Here's how the part is built. I have some questions about the finished solid (model axes, mm). A direction names the side the tool comes from. Round coordinates to 2 decimals unless told otherwise and drop trailing zeros. Order: outer loops, then holes, each group sorted by start corner. A loop starts at its lowest first (then second) coordinate and runs counter-clockwise, first axis right, second up. Notation, with made-up numbers: (-25, 47.5) - (29, 47.5) arc R22 cw to (29, 75.5) - close; hole circle Ø1 at (56.5, -38). An arc over 180 degrees is marked (long way). Answer as a JSON object with one key per item and string values.
```python
from build123d import *

# Parameters (mm, degrees)
BOSS_EXTRUDE1_DEPTH        = 100
CHAMFER1_SIZE              = 0.5
SKETCH5_R                  = 2
CUT_EXTRUDE1_DEPTH         = 200
CHAMFER2_SIZE              = 0.5
LPATTERN1_COUNT            = 3
LPATTERN1_PITCH            = 35
CHAMFER2_OF_LPATTERN1_SIZE = 0.5
CUT_EXTRUDE2_DEPTH         = 10
CUT_EXTRUDE2_DEPTH_BACK    = 10
SKETCH6_W                  = 15
SKETCH6_H                  = 40


with BuildPart() as part:
    # Sketch1 → Boss-Extrude1 (new body)
    with BuildSketch(Plane.XY):
        with BuildLine():
            Line((-3, 2), (-5, 2))
            Line((-5, 2), (-5, -2))
            Line((-5, -2), (5, -2))
            Line((5, -2), (5, 2))
            Line((5, 2), (3, 2))
            Line((3, 2), (3, 1.25))
            ThreePointArc((3, 1.25), (3.530330086, 1.030330086), (3.75, 0.5))
            ThreePointArc((3.75, 0.5), (3.530330086, -0.030330086), (3, -0.25))
            Line((3, -0.25), (3, -1))
            Line((3, -1), (-3, -1))
            Line((-3, -1), (-3, -0.25))
            ThreePointArc((-3, -0.25), (-3.75, 0.5), (-3, 1.25))
            Line((-3, 1.25), (-3, 2))
        make_face()
    extrude(amount=BOSS_EXTRUDE1_DEPTH)

    # Chamfer1
    chamfer1_edges = [part.edges().sort_by_distance(p)[0] for p in [
        (-3, -1, 50),
        (3, -1, 50),
        (5, 2, 50),
        (5, -2, 50),
        (-5, -2, 50),
        (-5, 2, 50),
    ]]
    chamfer(chamfer1_edges, length=CHAMFER1_SIZE)

    # Sketch5 → Cut-Extrude1 (cut)
    with BuildSketch(Plane(origin=(0, -1, 0), x_dir=(1, 0, 0), z_dir=(0, 1, 0))):
        with Locations(Location((0, -10, 0), (0, 0, 270))):
            Circle(SKETCH5_R)
        with Locations(Location((0, -20, 0), (0, 0, 270))):
            Circle(SKETCH5_R)
    cut_extrude1 = extrude(amount=-CUT_EXTRUDE1_DEPTH, mode=Mode.SUBTRACT)

    # Chamfer2
    chamfer2_edges = [part.edges().sort_by_distance(p)[0] for p in [
        (0, -1, 8),
        (0, -1, 18),
    ]]
    chamfer(chamfer2_edges, length=CHAMFER2_SIZE - 0.0001)  # a hair under: the kernel refuses the full size

    # LPattern1: Cut-Extrude1 ×3
    with Locations(*[(0, 0, i * LPATTERN1_PITCH) for i in range(1, LPATTERN1_COUNT)]):
        add(cut_extrude1, mode=Mode.SUBTRACT)

    # Chamfer2 of LPattern1
    chamfer2_of_lpattern1_edges = [part.edges().sort_by_distance(p)[0] for p in [
        (0, -1, 43),
        (0, -1, 53),
        (0, -1, 78),
        (0, -1, 88),
    ]]
    chamfer(chamfer2_of_lpattern1_edges, length=CHAMFER2_OF_LPATTERN1_SIZE - 0.0001)  # a hair under: the kernel refuses the full size

    # Sketch6 → Cut-Extrude2 (cut, two sides: drawn at the far end of the back side and taken through both)
    with BuildSketch(Plane(origin=(0, 0, 0), x_dir=(1, 0, 0), z_dir=(0, 1, 0)).offset(-CUT_EXTRUDE2_DEPTH_BACK)):
        with Locations((0, -80)):
            Rectangle(SKETCH6_W, SKETCH6_H)
    extrude(amount=CUT_EXTRUDE2_DEPTH + CUT_EXTRUDE2_DEPTH_BACK, mode=Mode.SUBTRACT)


solid = part.part
```
1. Imagine slicing it at C-C (z = 50). List the corners of the cut face in (x, y) for me.
Responses:
{"outline": "(-5, -1.5) - (-4.5, -2) - (4.5, -2) - (5, -1.5) - (5, 1.5) - (4.5, 2) - (3, 2) - (3, 1.25) arc R0.75 cw to (3, -0.25) - (3, -0.5) - (2.5, -1) - (-2.5, -1) - (-3, -0.5) - (-3, -0.25) arc R0.75 cw to (-3, 1.25) - (-3, 2) - (-4.5, 2) - (-5, 1.5) - close"}
2. If I drill on L1, parallel to X at y = 0.4, z = 42.5; L2, parallel to Y at x = 1.5, z = 51; L3, parallel to X at y = 1.1, z = 11, over which ranges is the centre line in solid material (lowest first)? Write a range as [from, to].
Responses:
{"L1": "[-5, -3.74], [3.74, 5]", "L2": "[-2, -1]", "L3": "[-5, -3.45], [3.45, 5]"}
3. Thinking about a two-plate mould opening in X: for faces 4 (the face through (0.601, -1.746, 56.908)), 5 (the face through (-0.1, -1.4, 60)), 6 (the face through (-0.766, -1.746, 46.847)), 7 (the face through (5, 0, 30)), which applies, pulls with the +X half, pulls with the -X half, needs draft (parallel to the pull), parting line crosses it, or undercut?
Responses:
{"face 4": "undercut", "face 5": "needs draft", "face 6": "undercut", "face 7": "pulls with the +X half"}
4. For faces 1 (the face through (4, 2, 30)), 2 (the face through (0, -1, 30)), 3 (the face through (-3.75, 0.48, 29.58)), which set-ups out of +Z, -Z, +X, -X, +Y, -Y let a thin tool reach every point of the face, with its end or its side?
Responses:
{"face 1": "+Z, -Z, +X, -X, +Y", "face 2": "+Z, -Z, +Y", "face 3": "+Z, -Z"}
5. For P1, Ø2.5, axis at x = 0, z = 10, coming from the +Y side; P2, Ø4, axis at x = 0, z = 23, coming from the +Y side, each with a flat end and sliding along its axis, tell me the tip position at first contact or that it passes through.
Responses:
{"P1": "through", "P2": "y = -1"}
6. Imagine slicing it at A-A (x = 0). List the corners of the cut face in (y, z) for me.
Responses:
{"outline": "(-2, 0) - (-1, 0) - (-1, 7.5) - (-1.5, 8) - (-2, 8) - close; (-2, 12) - (-1.5, 12) - (-1, 12.5) - (-1, 17.5) - (-1.5, 18) - (-2, 18) - close; (-2, 22) - (-1.5, 22) - (-1, 22.5) - (-1, 42.5) - (-1.5, 43) - (-2, 43) - close; (-2, 47) - (-1.5, 47) - (-1, 47.5) - (-1, 52.5) - (-1.5, 53) - (-2, 53) - close; (-2, 57) - (-1.5, 57) - (-1, 57.5) - (-1, 60) - (-2, 60) - close"}
